Could you check a few things on this model? Use its own coordinates, in mm. A direction names the side the tool comes from. Give positions to 0.01 mm unless a question says otherwise; leave off trailing zeros. Order: outer loops, then holes, each group sorted by start corner. A loop starts at its lowest first (then second) coordinate and runs counter-clockwise, first axis right, second up. Notation, with made-up numbers: M 48.25,21.5 L 85.25,21.5 A16 ccw 85.25,47.5 Z; hole C 11,88 d1. An arc over 180 degrees is marked long. Answer in a Markdown table with one row per item. Add a question column.
```python
from build123d import *

# Parameters (mm, degrees)
BASE_FLANGE1_DEPTH      = 100
EDGE_FLANGE1_DEPTH      = 100
EDGE_FLANGE1_BEND_DEPTH = 100
SKETCH8_W               = 99.3268
SKETCH8_H               = 0.7366
BOSS_EXTRUDE1_DEPTH     = 15


# Sheet-metal steps are written as plain solids
with BuildPart() as part:
    # Sketch1 → Base-Flange1 (new body)
    with BuildSketch(Plane(origin=(0, 0, 0), x_dir=(1, 0, 0), z_dir=(0, 1, 0))):
        with BuildLine():
            Line((-100, 132), (-0.7366, 132))
            ThreePointArc((-0.7366, 132), (-0.215745145, 131.784254855), (0, 131.2634))
            Line((0, 131.2634), (0, 0.7366))
            ThreePointArc((0, 0.7366), (-0.215745145, 0.215745145), (-0.7366, 0))
            Line((-0.7366, 0), (-100, 0))
            Line((-100, 0), (-100, -0.7366))
            Line((-100, -0.7366), (-0.7366, -0.7366))
            ThreePointArc((-0.7366, -0.7366), (0.30510971, -0.30510971), (0.7366, 0.7366))
            Line((0.7366, 0.7366), (0.7366, 131.2634))
            ThreePointArc((0.7366, 131.2634), (0.30510971, 132.30510971), (-0.7366, 132.7366))
            Line((-0.7366, 132.7366), (-100, 132.7366))
            Line((-100, 132.7366), (-100, 132))
        make_face()
    extrude(amount=BASE_FLANGE1_DEPTH)

    # Edge-Flange1 section (across the edge) → Edge-Flange1 (add)
    with BuildSketch(Plane(origin=(-100.8, 100, -132), x_dir=(1, 0, 0), z_dir=(0, -1, 0))):
        with BuildLine():
            Line((-0.7366, 0.7366), (-0.7366, 14.2634))
            Line((-0.7366, 14.2634), (0, 14.2634))
            Line((0, 14.2634), (0, 0.7366))
            ThreePointArc((0, 0.7366), (0.215745145, 0.215745145), (0.7366, 0))
            Line((0.7366, 0), (0.8, 0))
            Line((0.8, 0), (0.8, -0.7366))
            Line((0.8, -0.7366), (0.7366, -0.7366))
            ThreePointArc((0.7366, -0.7366), (-0.30510971, -0.30510971), (-0.7366, 0.7366))
        make_face()
    extrude(amount=EDGE_FLANGE1_DEPTH)

    # Edge-Flange1 section 2 (across the edge) → Edge-Flange1 bend (add)
    with BuildSketch(Plane(origin=(-100.8, 0, 0), x_dir=(1, 0, 0), z_dir=(0, 1, 0))):
        with BuildLine():
            Line((-0.7366, 0.7366), (-0.7366, 14.2634))
            Line((-0.7366, 14.2634), (0, 14.2634))
            Line((0, 14.2634), (0, 0.7366))
            ThreePointArc((0, 0.7366), (0.215745145, 0.215745145), (0.7366, 0))
            Line((0.7366, 0), (0.8, 0))
            Line((0.8, 0), (0.8, -0.7366))
            Line((0.8, -0.7366), (0.7366, -0.7366))
            ThreePointArc((0.7366, -0.7366), (-0.30510971, -0.30510971), (-0.7366, 0.7366))
        make_face()
    extrude(amount=EDGE_FLANGE1_BEND_DEPTH)

    # Sketch8 → Boss-Extrude1 (add)
    with BuildSketch(Plane(origin=(0, 100, 0), x_dir=(1, 0, 0), z_dir=(0, 1, 0))):
        with Locations((-50.4, -0.3683)):
            Rectangle(SKETCH8_W, SKETCH8_H)
        with Locations((-50.4, 132.3683)):
            Rectangle(SKETCH8_W, SKETCH8_H)
    extrude(amount=BOSS_EXTRUDE1_DEPTH)


solid = part.part
```
1. Suppose I cut it at C-C on y = 97.5. List the corners of the cut face in (x, z) for me, plus the area to 3 significant figures.
2. Suppose I cut it at B-B on x = -48.5. List the corners of the cut face in (y, z) for me.
3. Thinking about a two-plate mould opening in X: for faces 3 (the flat face through (-51, 58, -132)), 4 (the flat face through (0.737, 49, -65)), 5 (the flat face through (-50, 58, -132.737)), which applies, pulls with the +X half, pulls with the -X half, needs draft (parallel to the pull), parting line crosses it, or undercut?
4. Suppose I cut it at D-D on z = -42. List the corners of the cut face in (x, y) for me, plus the area to 3 significant figures.
5. If I drill on line 1 along Z through (x, y) = (-11.5, 85); line 2 along X through (y, z) = (96, -120); line 3 along X through (y, z) = (75, -31), over which ranges is the centre line in solid material (lowest first)? Write a range as [from, to].
6. For faces 1 (the flat face through (0, 49, -67)), 2 (the flat face through (-101.537, 51, -125)), which set-ups out of +Z, -Z, +X, -X, +Y, -Y let a thin tool reach every point of the face, with its end or its side?
7. Suppose I cut it at A-A on z = -8.5. List the corners of the cut face in (x, y) for me, plus the area to 3 significant figures.
8. Will these pins go through, and if not, where does the flat tip stop? P1, Ø0.6, axis at y = 104.5, z = 0.5, coming from the +X side; P2, Ø0.7, axis at x = -101, z = -6, coming from the +Y side; P3, Ø0.6, axis at x = -101.5, y = 49.5, coming from the -Z side.
Findings below:
| question | item | result |
|---|---|---|
| 1 | outline | M -101.54,-131.26 A1.47 ccw -100.06,-132.74 L -0.74,-132.74 A1.47 ccw 0.74,-131.26 L 0.74,-0.74 A1.47 ccw -0.74,0.74 L -100.06,0.74 A1.47 ccw -101.54,-0.74 L -101.54,-14.26 L -100.8,-14.26 L -100.8,-0.74 A0.74 cw -100.06,0 L -0.74,0 A0.74 cw 0,-0.74 L 0,-131.26 A0.74 cw -0.74,-132 L -100.06,-132 A0.74 cw -100.8,-131.26 L -100.8,-117.74 L -101.54,-117.74 Z |
| 1 | area | 268 mm2 |
| 2 | outline | M 0,-132.74 L 115,-132.74 L 115,-132 L 0,-132 Z; M 0,0 L 115,0 L 115,0.74 L 0,0.74 Z |
| 3 | face 3 | undercut |
| 3 | face 4 | pulls with the +X half |
| 3 | face 5 | needs draft |
| 4 | outline | M 0,0 L 0.74,0 L 0.74,100 L 0,100 Z |
| 4 | area | 73.7 mm2 |
| 5 | line 1 | [-132.74, -132], [0, 0.74] |
| 5 | line 2 | [-101.54, -100.8], [0, 0.74] |
| 5 | line 3 | [0, 0.74] |
| 6 | face 1 | +Y, -Y |
| 6 | face 2 | +Z, -Z, -X, +Y, -Y |
| 7 | outline | M -101.54,0 L -100.8,0 L -100.8,100 L -101.54,100 Z; M 0,0 L 0.74,0 L 0.74,100 L 0,100 Z |
| 7 | area | 147 mm2 |
| 8 | P1 | x = -0.74 |
| 8 | P2 | y = 100 |
| 8 | P3 | z = -132.2 |
